Read the model definition and answer for the solid it produces. Units are mm, in the model's axes. Face numbers are marked on the shaded views. A direction names the side the tool comes from. Give positions to 0.01 mm unless a question says otherwise; leave off trailing zeros. Write each loop counter-clockwise with the first axis right and the second up, starting at its lowest first coordinate (ties: lowest second). Pieces come first, ordered by that corner, then holes.
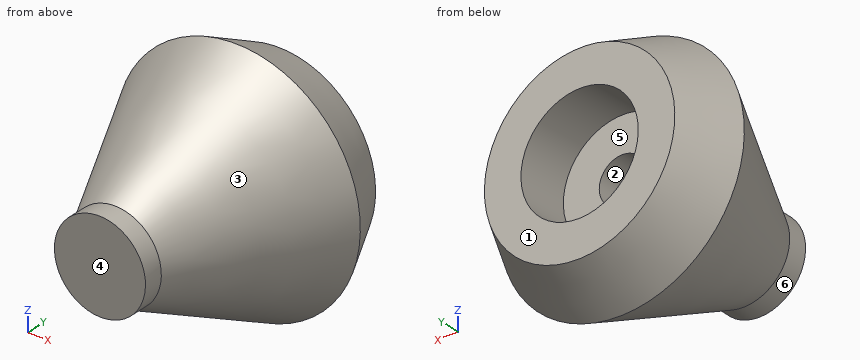
Autodesk Inventor part; units mm, degrees
ref_plane "YZ Plane" through (0, 0, 0) normal (1, 0, 0) x (0, 1, 0)
ref_plane "XZ Plane" through (0, 0, 0) normal (0, 1, 0) x (-1, 0, 0)
ref_plane "XY Plane" through (0, 0, 0) normal (0, 0, 1) x (1, 0, 0)
sketch "Sketch1" plane through (0, 0, 0) normal (1, 0, 0) x (0, 1, 0)
  line L0 (1.947, 4.4699) -> (0, 4.4699)
  line L1 (0, 4.4699) -> (0, 0)
  line L2 (0, 0) -> (1.947, 0)
  line L3 (1.947, 0) -> (1.947, 4.4699)
sketch "Sketch2" plane through (0, 0, 0) normal (1, 0, 0) x (0, 1, 0)
  line L0 (1.947, 0) -> (1.947, 4.4699)
  line L1 (0, 0) -> (1.947, 0)
  line L2 (1.947, 4.4699) -> (0, 4.4699)
  line L3 (16.9602, -1.2877) -> (22.1681, -1.2877)
  line L4 (22.1681, -1.2877) -> (22.1681, -4.8754)
  line L5 (22.1681, -4.8754) -> (16.9602, -7.5373)
  line L6 (16.9602, -7.5373) -> (1.947, 0)
  line L7 (1.947, 2.235) -> (16.9602, 2.235)
  line L8 (16.9602, 2.235) -> (16.9602, -1.2877)
  line L9 (1.947, 4.4699) -> (5.6822, 4.4699)
sketch "Sketch3" plane through (0, 0, 0) normal (1, 0, 0) x (0, 1, 0)
  point P0 (0, 0)
revolve "Revolution1" add sketch "Sketch2" angle 360 about axis through (0, 1.947, 4.4699) along (0, 1, 0)
revolve "Revolution2" add sketch "Sketch1" angle 360 about axis through (0, 1.947, 4.4699) along (0, -1, 0)
properties part number "Train smoke stack" material "ABS Plastic"
Item 1: Section A-A (x = 0) is taken. Write down the section's boundary in (y, z) (1 decimal).
Result set:
outline: (0, 0) - (1.9, 0) - (17, -7.5) - (22.2, -4.9) - (22.2, -1.3) - (17, -1.3) - (17, 2.2) - (1.9, 2.2) - (1.9, 6.7) - (17, 6.7) - (17, 10.2) - (22.2, 10.2) - (22.2, 13.8) - (17, 16.5) - (1.9, 8.9) - (0, 8.9) - close
Item 2: Section B-B (y = 4.25) is taken. Write down the section's boundary in (x, z) (3 decimals).
Result set:
outline: circle Ø11.252 at (0, 4.47); hole circle Ø4.47 at (0, 4.47)
Item 3: Which of the six approach directions +Z, -Z, +X, -X, +Y, -Y give full straight-line access (tool end or side, diameter ignored) to the marked faces 4, 5 and 6?
Result set:
face 4: +Z, -Z, +X, -X, -Y
face 5: +Y
face 6: -Y
Item 4: Section C-C (y = 12.5) is taken. Write down the section's boundary in (x, z) (3 decimals), and give its area (3 significant figures).
Result set:
outline: circle Ø19.536 at (0, 4.47); hole circle Ø4.47 at (0, 4.47)
area: 284 mm2
Item 5: Determine the mould class of the marked faces 1, 2 and 3 for opening direction X: pulls with the +X half, pulls with the -X half, needs draft (parallel to the pull), parting line crosses it, or undercut.
Result set:
face 1: needs draft
face 2: undercut
face 3: parting line crosses it
Item 6: Find the intervals of material crossed by line 1 along Y through (x, z) = (2.75, 2.5); line 2 along Z through (x, y) = (0, 19.4); line 3 along Z through (x, y) = (0, 9.25) (3 decimals), in increasing order.
Result set:
line 1: y = 0 to 16.96
line 2: z = -6.29 to -1.29, 10.23 to 15.23
line 3: z = -3.666 to 2.235, 6.705 to 12.606
Item 7: Each of these flat-tipped pins is pushed along its axis until it touches: pin 1 Ø3.5 at (x, z) = (0, 4.5) entering from +Y; pin 2 Ø12 at (x, y) = (-1, 4.5) entering from -Z; pin 3 Ø3 at (x, y) = (-1.5, 4) entering from +Z; pin 4 Ø5 at (x, z) = (1.5, 14) entering from +Y. Where does it stop, or does it pass through?
Result set:
pin 1: stops at y = 1.95
pin 2: stops at z = -4.27
pin 3: stops at z = 10.6
pin 4: stops at y = 22.17
